from build123d import *

# Parameters (mm, degrees)
AUFSATZ_LINEAR_AUSTRAGEN1_DEPTH = 16
SKIZZE2_W                       = 1900
SKIZZE2_H                       = 60
SCHNITT_LINEAR_AUSTRAGEN1_DEPTH = 2371.707911152


with BuildPart() as part:
    # Skizze1 → Aufsatz-Linear austragen1 (new body)
    with BuildSketch(Plane(origin=(0, 0, 0), x_dir=(1, 0, 0), z_dir=(0, 1, 0))):
        with BuildLine():
            Line((2100, 0), (2100, 1100))
            Line((2100, 1100), (1800, 1100))
            Line((1800, 1100), (1800, 700))
            ThreePointArc((1800, 700), (1756.066017178, 593.933982822), (1650, 550))
            Line((1650, 550), (0, 550))
            Line((0, 550), (0, 0))
            Line((0, 0), (2100, 0))
        make_face()
    extrude(amount=AUFSATZ_LINEAR_AUSTRAGEN1_DEPTH)

    # Skizze2 → Schnitt-Linear austragen1 (cut, through all)
    with BuildSketch(Plane(origin=(0, 16, 0), x_dir=(1, 0, 0), z_dir=(0, 1, 0))):
        with Locations((1000, 30)):
            Rectangle(SKIZZE2_W, SKIZZE2_H)
    extrude(amount=-SCHNITT_LINEAR_AUSTRAGEN1_DEPTH, mode=Mode.SUBTRACT)


solid = part.part
The model under review builds one solid part; all positions refer to its coordinate system, in mm. Coordinates: 2 decimals unless noted, no trailing zeros. Write each loop counter-clockwise with the first axis right and the second up, starting at its lowest first coordinate (ties: lowest second). Pieces come first, ordered by that corner, then holes. Notation, with made-up numbers: M 38,75.5 L 53,75.5 A7 ccw 53,82.5 Z; hole C -28,32.5 d9. An arc over 180 degrees is marked long. Put each result on its own line as item: value.
1) Clearance check with flat-ended pins moving along their axes: pin 1 Ø8 at (x, y) = (906, 7) entering from -Z; pin 2 Ø2 at (x, y) = (218.5, 5.5) entering from +Z. State where each tip first meets the part, or that it passes through.
Computed:
pin 1: stops at z = -550
pin 2: stops at z = -60
2) Add section C-C on z = -737.5. Give the boundary of the cut face in (x, y).
Computed:
outline: M 1800,0 L 2100,0 L 2100,16 L 1800,16 Z
3) Wall thickness on probe 1 along Z at (x, y) = (1388.5, 12.5); probe 2 along X at (y, z) = (2.25, -824); probe 3 along X at (y, z) = (4.5, -644.5): over which ranges is each line inside the solid? List them lowest first. Write a range as [from, to].
Computed:
probe 1: z = [-550, -60]
probe 2: x = [1800, 2100]
probe 3: x = [1789.35, 2100]
4) Add section A-A on y = 13.25. Give the boundary of the cut face in (x, z), then the cut area to 3 significant figures.
Computed:
outline: M 0,-550 L 1650,-550 A150 cw 1800,-700 L 1800,-1100 L 2100,-1100 L 2100,0 L 1950,0 L 1950,-60 L 50,-60 L 50,0 L 0,0 Z
area: 1,210,000 mm2
5) Add section B-B on x = 1828. Give the boundary of the cut face in (y, z).
Computed:
outline: M 0,-1100 L 16,-1100 L 16,-60 L 0,-60 Z
